Build history of the part. All positions in model axes, mm. A direction names the side the tool comes from. Round coordinates to 2 decimals unless told otherwise and drop trailing zeros. Order: outer loops, then holes, each group sorted by start corner. A loop starts at its lowest first (then second) coordinate and runs counter-clockwise, first axis right, second up. Notation, with made-up numbers: (36.25, 54.5) -> (62.25, 54.5) arc R23 cw to (62.25, 93.5) -> close; hole circle Ø2 at (66.5, -40). An arc over 180 degrees is marked (long way). Answer as a JSON object with one key per item and string values.
Autodesk Inventor part; units mm, degrees
ref_plane "YZ Plane" through (0, 0, 0) normal (1, 0, 0) x (0, 1, 0)
ref_plane "XZ Plane" through (0, 0, 0) normal (0, 1, 0) x (-1, 0, 0)
ref_plane "XY Plane" through (0, 0, 0) normal (0, 0, 1) x (1, 0, 0)
sketch "Sketch1" plane through (0, 0, 0) normal (0, 0, 1) x (1, 0, 0)
  line L0 (-123.35, 77) -> (123.35, 77)
  line L1 (123.35, 77) -> (123.35, -77)
  line L2 (123.35, -77) -> (-123.35, -77)
  line L3 (-123.35, -77) -> (-123.35, 77)
  point P0 (0, 0)
  point P1 (-123.35, 0)
  point P2 (0, 77)
  dimension "d0" = 246.7
  dimension "d1" = 154
extrude "Extrusion1" add sketch "Sketch1" along normal blind 15
sketch "Sketch2" plane through (0, 0, 15) normal (0, 0, 1) x (1, 0, 0)
  line L0 (-123.35, 77) -> (123.35, 77)
  line L1 (123.35, 77) -> (123.35, -77)
  line L2 (62.65, 77) -> (62.65, 28.2)
  line L3 (62.65, 28.2) -> (123.35, 28.2)
  line L4 (123.35, -77) -> (-123.35, -77)
  line L5 (62.65, 58.2) -> (92.65, 28.2)
  dimension "d4" = 60.7
  dimension "d5" = 105.2
  dimension "d6" = 45
  dimension "d7" = 30.7
extrude "Extrusion2" cut sketch "Sketch2" against normal through all contours L0 L1 L3 L5 L2
sketch "Sketch3" plane through (0, 0, 15) normal (0, 0, 1) x (1, 0, 0)
  line L0 (123.35, 28.2) -> (123.35, -77)
  line L1 (123.35, -42.45) -> (92.65, -42.45)
  line L2 (92.65, -42.45) -> (71.05, -64.05)
  line L3 (71.05, -64.05) -> (71.05, -77)
  line L4 (123.35, -77) -> (-123.35, -77)
  point P0 (92.65, 28.2)
  point P1 (62.65, 58.2)
  dimension "d10" = 34.55
  dimension "d11" = 45
  dimension "d41" = 52.3
extrude "Extrusion3" cut sketch "Sketch3" against normal through all
fillet "Fillet1" radius 6.35 4 edges at (62.65, 58.2, 7.5) (92.65, 28.2, 7.5) (92.65, -42.45, 7.5) (71.05, -64.05, 7.5)
sketch "Sketch4" plane through (0, 0, 15) normal (0, 0, 1) x (1, 0, 0)
  line L0 (-123.35, 77) -> (-103.35, 77)
  line L1 (-103.35, 77) -> (-103.35, 40)
  line L2 (-103.35, 40) -> (-123.35, 40)
  line L3 (-123.35, 40) -> (-123.35, 77)
  dimension "d15" = 37
  dimension "d16" = 20
extrude "Extrusion4" add sketch "Sketch4" along normal blind 1
sketch "Sketch5" plane through (0, 0, 16) normal (0, 0, 1) x (1, 0, 0)
  line L0 (-119.35, 55.5) -> (-119.35, 61.5)
  arc A0 (-107.35, 61.5) -> (-119.35, 61.5) centre (-113.35, 61.5) ccw
  line L1 (-107.35, 61.5) -> (-107.35, 55.5)
  arc A1 (-119.35, 55.5) -> (-107.35, 55.5) centre (-113.35, 55.5) ccw
  line L2 (-119.35, 58.5) -> (-107.35, 58.5) construction
  line L3 (-103.35, 77) -> (-103.35, 40) construction
  line L4 (-103.35, 40) -> (-123.35, 40) construction
  point P0 (-103.35, 58.5)
  point P1 (-113.35, 40)
  point P2 (-113.35, 58.5)
  dimension "d23" = 12
  dimension "d24" = 18
extrude "Extrusion5" cut sketch "Sketch5" against normal through all
pattern_linear "Rectangular Pattern1" count 2 spacing 118 along (1, 0, 0) of "Extrusion4", "Extrusion5"
sketch "Sketch6" plane through (0, 0, 15) normal (0, 0, 1) x (1, 0, 0)
  line L0 (-123.35, -77) -> (-103.35, -77)
  line L1 (-103.35, -77) -> (-103.35, -44.4)
  line L2 (-103.35, -44.4) -> (-123.35, -44.4)
  line L3 (-123.35, -44.4) -> (-123.35, -77)
  point P0 (-103.35, 40)
  dimension "d30" = 32.6
extrude "Extrusion6" add sketch "Sketch6" along normal blind 1
sketch "Sketch7" plane through (0, -119.2, 16) normal (0, 0, 1) x (1, 0, 0)
  line L0 (-119.35, 55.5) -> (-119.35, 61.5)
  arc A0 (-107.35, 61.5) -> (-119.35, 61.5) centre (-113.35, 61.5) ccw
  line L1 (-107.35, 61.5) -> (-107.35, 55.5)
  arc A1 (-119.35, 55.5) -> (-107.35, 55.5) centre (-113.35, 55.5) ccw
  line L2 (-119.35, 58.5) -> (-107.35, 58.5) construction
  line L3 (-103.35, 77) -> (-103.35, 40) construction
  line L4 (-103.35, 40) -> (-123.35, 40) construction
  point P0 (-103.35, 58.5)
  point P1 (-113.35, 40)
  point P2 (-113.35, 58.5)
  dimension "d34" = 12
  dimension "d33" = 18
extrude "Extrusion7" cut sketch "Sketch7" against normal through all
pattern_linear "Rectangular Pattern2" count 2 spacing 166 along (1, 0, 0) of "Extrusion7", "Extrusion6"
hole "Hole1" at (-105.35, -22.45, 15) direction (0, 0, -1) diameter 8.8 end through all counterbore diameter 15 counterbore depth 9
pattern_linear "Rectangular Pattern3" count 2 spacing 39.13 along (0, 1, 0) count 2 spacing 219.2 along (1, 0, 0) of "Hole1"
properties part number "VERTICAL PLATE" material "Steel, Mild"
1) Which spindle directions (+Z, -Z, +X, -X, +Y, -Y) get a long thin tool onto all of the face, cutting with end or side? Do faces 1 (the face through (63.147, 58.368, 7.395)), 2 (the face through (52.8, -51.7, 8.1)), 3 (the face through (-102, 13, 6)). Say none if no direction does.
Checked values:
{"face 1": "+Z, -Z, +X, +Y", "face 2": "+Z, -Z", "face 3": "+Z"}
2) Cut at A-A, the plane y = 16.68. Give the cut face in (x, z).
Checked values:
{"outline": "(-123.35, 0) -> (-109.75, 0) -> (-109.75, 6) -> (-112.85, 6) -> (-112.85, 15) -> (-123.35, 15) -> close; (-100.95, 0) -> (109.45, 0) -> (109.45, 6) -> (106.35, 6) -> (106.35, 15) -> (-97.85, 15) -> (-97.85, 6) -> (-100.95, 6) -> close; (118.25, 0) -> (123.35, 0) -> (123.35, 15) -> (121.35, 15) -> (121.35, 6) -> (118.25, 6) -> close"}
3) Cut at B-B, the plane x = 4.65. Give the cut face in (y, z).
Checked values:
{"outline": "(-77, 0) -> (49.5, 0) -> (49.5, 16) -> (40, 16) -> (40, 15) -> (-77, 15) -> close; (67.5, 0) -> (77, 0) -> (77, 16) -> (67.5, 16) -> close"}
4) Cut at C-C, the plane z = 11.75. Count the separate pieces of the cut face and the enclosed holes in it, plus the area to 3 significant figures.
Checked values:
{"separate pieces": "1", "enclosed holes": "8", "area": "32,500 mm²"}
5) Pull direction Y, two halves, no side cores. Call faces 4 (the face through (62.65, 69, 8)), 5 (the face through (4.5, 49.5, 8.1)), 6 (the face through (-28, -77, 8)), 7 (the face through (-32, 77, 8)): pulls with the +Y half, pulls with the -Y half, needs draft (parallel to the pull), parting line crosses it, or undercut.
Checked values:
{"face 4": "needs draft", "face 5": "undercut", "face 6": "pulls with the -Y half", "face 7": "pulls with the +Y half"}
6) Cut at D-D, the plane x = 52.65. Give the cut face in (y, z), plus the area to 3 significant figures.
Checked values:
{"outline": "(-77, 0) -> (-69.7, 0) -> (-69.7, 16) -> (-77, 16) -> close; (-51.7, 0) -> (77, 0) -> (77, 15) -> (-44.4, 15) -> (-44.4, 16) -> (-51.7, 16) -> close", "area": "2,050 mm²"}
7) Probe L1, parallel to X at y = -22.45, z = 11; L2, parallel to Y at x = -105.35, z = 3.1; L3, parallel to X at y = -22.45, z = 2. List the from-to ranges inside material, lowest first. Write a range as from..to.
Checked values:
{"L1": "x = -123.35..-112.85, -97.85..106.35, 121.35..123.35", "L2": "y = -77..-26.85, -18.05..12.28, 21.08..77", "L3": "x = -123.35..-109.75, -100.95..109.45, 118.25..123.35"}
8) Flat gauge pins, fed straight in: pin 1 Ø7.5 at (x, y) = (113.5, 14.5) entering from +Z; pin 2 Ø7.5 at (x, z) = (105, 5) entering from -Y; pin 3 Ø2 at (x, z) = (68, 5) entering from +Y. Where does each tip first touch, or does it go through?
Checked values:
{"pin 1": "stops at z = 6", "pin 2": "stops at y = -42.45", "pin 3": "stops at y = 53.85"}
